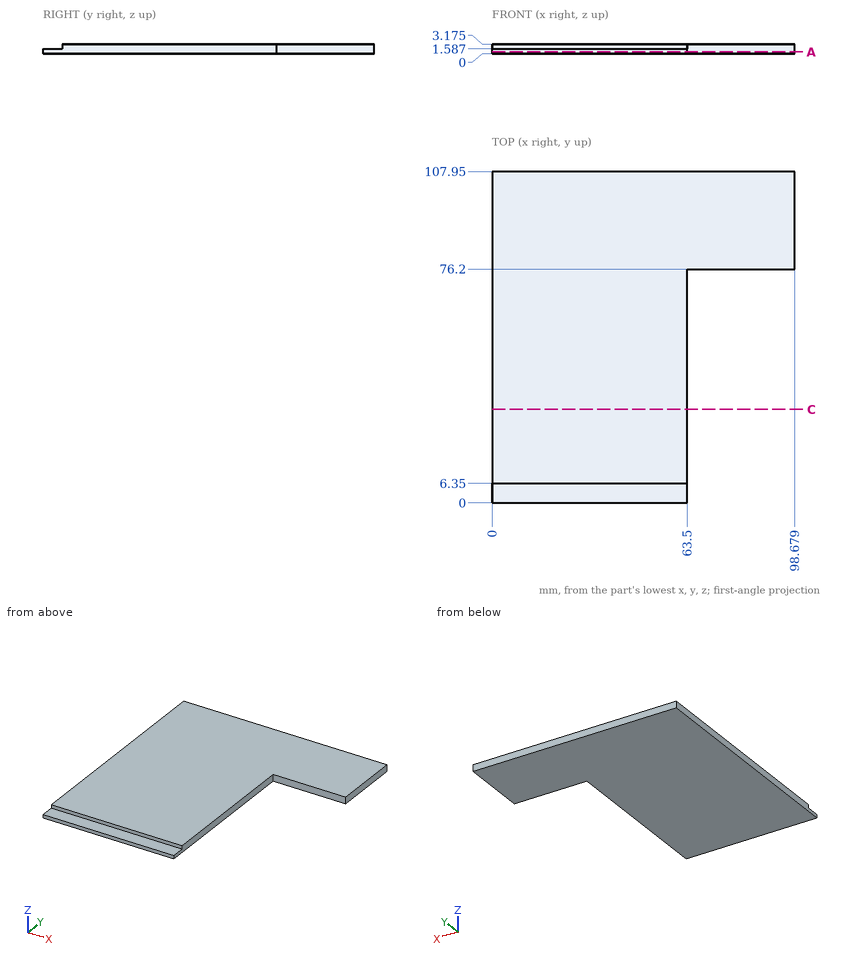
Part print with two shaded views. Sizes in mm from the minimum x, y, z corner. Round coordinates to 2 decimals unless told otherwise and drop trailing zeros. Loops run counter-clockwise (first coordinate to the right, second up) from the corner with the lowest first, then second, coordinate; pieces in that order, holes last.
Item 1: Saw through at A-A (z = 0.6). List the corners of the cut face in (x, y).
Item 2: Drill centre lines: line 1 along Y through (x, z) = (50.5, 2.1); line 2 along X through (y, z) = (9.5, 2); line 3 along Y through (x, z) = (72.5, 1.05). Where is each one in solid material? Low to high.
Item 3: Pin check, flat tips, straight feed: P1, Ø1.6, axis at x = 78, z = 1, coming from the -Y side; P2, Ø1.6, axis at y = 45, z = 1, coming from the +X side; P3, Ø8, axis at x = 17.5, y = 61, coming from the -Z side; P4, Ø1.9, axis at x = 31, y = 3.5, coming from the +Z side. Stop position of each tip, or through.
Item 4: Saw through at C-C (y = 30.5). List the corners of the cut face in (x, z) (1 decimal).
Worked answers:
1. outline: (0, 0) - (63.5, 0) - (63.5, 76.2) - (98.68, 76.2) - (98.68, 107.95) - (0, 107.95) - close
2. line 1: y = 6.35 to 107.95
2. line 2: x = 0 to 63.5
2. line 3: y = 76.2 to 107.95
3. P1: stops at y = 76.2
3. P2: stops at x = 63.5
3. P3: stops at z = 0
3. P4: stops at z = 1.59
4. outline: (0, 0) - (63.5, 0) - (63.5, 3.2) - (0, 3.2) - close
